Source: CAD feature listing. Evaluate the final solid. Frame: model axes, mm. Face numbers are marked on the shaded views. A direction names the side the tool comes from. Coordinates: 2 decimals unless noted, no trailing zeros. Order: outer loops, then holes, each group sorted by start corner. A loop starts at its lowest first (then second) coordinate and runs counter-clockwise, first axis right, second up.
Item 1: Section B-B on y = 19.5. Return the cut outline in (x, z).
Item 2: Section A-A on z = -22. Return the cut outline in (x, y).
Item 3: Reachability of the marked faces 1, 2 and 3 from +Z, -Z, +X, -X, +Y, -Y: full face, straight path, thin tool, end or side. Return the list, or none.
Item 4: Contact query for flat-ended pins moving along their axis: P1, Ø5, axis at y = 31.5, z = -61, coming from the -X side; P2, Ø0.5, axis at x = 82, z = -3.5, coming from the +Y side; P3, Ø0.6, axis at x = 22, z = -2.5, coming from the +Y side. Output: stop coordinate, or through.
Item 5: Ray query, line 1 (Z direction, x = 56, y = 2.5); line 2 (X direction, y = 64, z = -82). Return the intervals inside material, ascending.
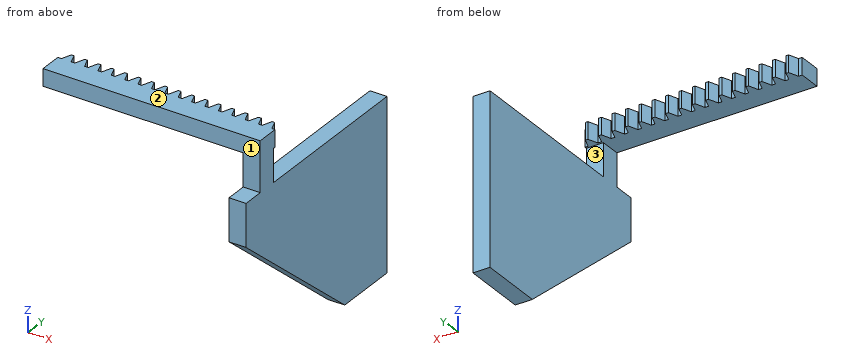
from build123d import *

# Parameters (mm, degrees)
BLANKSKE_W          = 120
BLANKSKE_H          = 16
BLANK_DEPTH         = 8
TOOTHCUTSIM_DEPTH   = 122.326007105
TEETHCUTS_COUNT     = 20
TEETHCUTS_PITCH     = 6.2831853
SKETCH1_W           = 8
SKETCH1_H           = 1
CUT_EXTRUDE1_DEPTH  = 122.326007105
BOSS_EXTRUDE2_DEPTH = 8
CUT_EXTRUDE2_DEPTH  = 183.738200713


with BuildPart() as part:
    # BlankSke → Blank (new body)
    with BuildSketch(Plane.XY):
        with Locations((60, 8)):
            Rectangle(BLANKSKE_W, BLANKSKE_H)
    extrude(amount=-BLANK_DEPTH)

    # TooCutSkeSim → ToothCutSim (cut, through all)
    with BuildSketch(Plane.XY):
        Polygon((0.861870739, 11.5), (-0.861870739, 11.5), (-2.508981637, 16.0254), (2.508981637, 16.0254), align=None)
    toothcutsim = extrude(amount=-TOOTHCUTSIM_DEPTH, mode=Mode.SUBTRACT)

    # TeethCuts: ToothCutSim ×20
    with Locations(*[(i * TEETHCUTS_PITCH, 0, 0) for i in range(1, TEETHCUTS_COUNT)]):
        add(toothcutsim, mode=Mode.SUBTRACT)

    # Sketch1 → Cut-Extrude1 (cut, through all)
    with BuildSketch(Plane(origin=(120, 0, 0), x_dir=(0, 0, -1), z_dir=(1, 0, 0))):
        with Locations((4, 0.5)):
            Rectangle(SKETCH1_W, SKETCH1_H)
    extrude(amount=-CUT_EXTRUDE1_DEPTH, mode=Mode.SUBTRACT)

    # Sketch2 → Boss-Extrude2 (add)
    with BuildSketch(Plane(origin=(120, 0, 0), x_dir=(0, 0, -1), z_dir=(1, 0, 0))):
        Polygon((8, 1), (23.5, 1), (23.5, -9), (43.5, -9), (103.5, 61), (103.5, 91), (23.5, 91), (23.5, 10.5), (8, 10.5), align=None)
    extrude(amount=-BOSS_EXTRUDE2_DEPTH)

    # Sketch3 → Cut-Extrude2 (cut, through all)
    with BuildSketch(Plane.XY):
        with BuildLine():
            Line((0, 1), (0, 11.5))
            ThreePointArc((0, 11.5), (0.43093537, 11.93093537), (0.861870739, 11.5))
            Line((0.861870739, 11.5), (2.499736794, 16))
            Line((2.499736794, 16), (3.783448506, 16))
            Line((3.783448506, 16), (5.421314561, 11.5))
            Line((5.421314561, 11.5), (7.145056039, 11.5))
            Line((7.145056039, 11.5), (8.782922094, 16))
            Line((8.782922094, 16), (10.066633806, 16))
            Line((10.066633806, 16), (11.704499861, 11.5))
            Line((11.704499861, 11.5), (13.428241339, 11.5))
            Line((13.428241339, 11.5), (15.066107394, 16))
            Line((15.066107394, 16), (15.70796325, 16))
            Line((15.70796325, 16), (16.349819106, 16))
            Line((16.349819106, 16), (17.987685161, 11.5))
            Line((17.987685161, 11.5), (17.987685161, 1))
            Line((17.987685161, 1), (15.70796325, 1))
            Line((15.70796325, 1), (6.161314561, 1))
            Line((6.161314561, 1), (0, 1))
        make_face()
    extrude(amount=-CUT_EXTRUDE2_DEPTH, mode=Mode.SUBTRACT)


solid = part.part
Answer list:
1. outline: (112, -67.93) - (120, -67.93) - (120, -23.5) - (112, -23.5) - close
2. outline: (112, 1) - (120, 1) - (120, 10.5) - (112, 10.5) - close
3. face 1: +Z, +X, -X, -Y
3. face 2: +Z, +X, -X, +Y, -Y
3. face 3: +X, -X, +Y
4. P1: stops at x = 112
4. P2: stops at y = 11.5
4. P3: stops at y = 16
5. line 1: z = -8 to 0
5. line 2: x = 112 to 120
